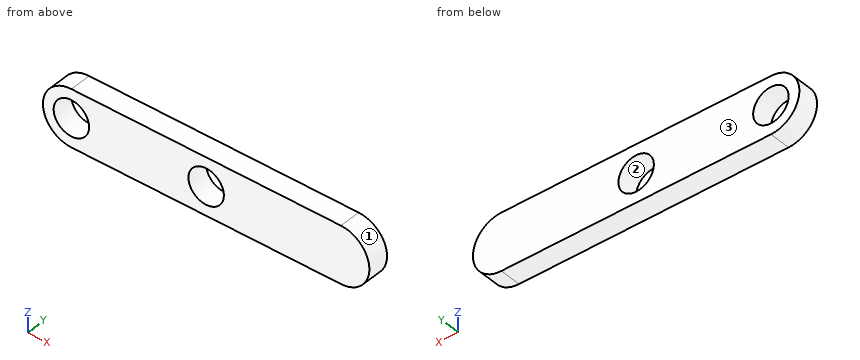
Autodesk Inventor part; units mm, degrees
ref_plane "YZ Plane" through (0, 0, 0) normal (1, 0, 0) x (0, 1, 0)
ref_plane "XZ Plane" through (0, 0, 0) normal (0, 1, 0) x (-1, 0, 0)
ref_plane "XY Plane" through (0, 0, 0) normal (0, 0, 1) x (1, 0, 0)
sketch "Sketch1" plane through (0, 0, 0) normal (0, 1, 0) x (-1, 0, 0)
  circle A0 centre (0, 0) radius 2.63
  line L0 (0, 0) -> (-2.63, 0) construction
  circle A1 centre (-20, 0) radius 2.63
  circle A2 centre (0, 0) radius 4.2175 construction
  circle A3 centre (-20, 0) radius 4.2175 construction
  line L1 (0, 4.2175) -> (-40, 4.2175)
  line L2 (0, -4.2175) -> (-40, -4.2175)
  arc A4 (-40, 4.2175) -> (-40, -4.2175) centre (-40, 0) ccw
  arc A5 (0, -4.2175) -> (0, 4.2175) centre (0, 0) ccw
  dimension "d0" = 5.26
  dimension "d1" = 20
  dimension "d2" = 1.5875
  dimension "d3" = 20
extrude "Extrusion1" add sketch "Sketch1" along normal blind 3.175
properties part number "CNC-011-XAxisHardStop" material "Aluminum 6061"
The listing builds one solid part. Answer for the finished solid, in the listing's coordinates (mm). Face numbers are marked on the shaded views. Round coordinates to 2 decimals unless told otherwise and drop trailing zeros. Loops run counter-clockwise (first coordinate to the right, second up) from the corner with the lowest first, then second, coordinate; pieces in that order, holes last. Notation, with made-up numbers: (-33, 84.5) - (10, 84.5) arc R11 cw to (10, 97.5) - close; hole circle Ø2 at (79.5, -31.75). An arc over 180 degrees is marked (long way). Return JSON: item names as keys, results as strings. Group by question number.
1. The part is cut by section A-A on x = 20. Determine the outline of the cut face in (y, z) (1 decimal).
2. The mould has two halves that part along Z. Classify the marked faces 1, 2 and 3: pulls with the +Z half, pulls with the -Z half, needs draft (parallel to the pull), parting line crosses it, or undercut.
3. This flat-tipped pin is pushed along its axis until it touches: P1, Ø1.5, axis at x = 14.5, z = 3, coming from the -Y side. Where does it stop, or does it pass through?
4. The part is cut by section D-D on z = -2. Determine the outline of the cut face in (x, y) (3 decimals).
5. The part is cut by section C-C on z = 1. Determine the outline of the cut face in (x, y) (3 decimals), then the cut area to 3 significant figures.
6. The part is cut by section B-B on y = 2.5. Determine the outline of the cut face in (x, z) (1 decimal).
7. Consider probe 1 along Z at (x, y) = (20, 1.2); probe 2 along X at (y, z) = (1.6, 0.75); probe 3 along X at (y, z) = (2.7, -1). Determine where each line is inside the solid, lowest interval first.
Resolved:
{
 "1": {"outline": "(0, -4.2) - (3.2, -4.2) - (3.2, -2.6) - (0, -2.6) - close; (0, 2.6) - (3.2, 2.6) - (3.2, 4.2) - (0, 4.2) - close"},
 "2": {"face 1": "parting line crosses it", "face 2": "undercut", "face 3": "needs draft"},
 "3": {"P1": "stops at y = 0"},
 "4": {"outline": "(-3.713, 0) - (-1.708, 0) - (-1.708, 3.175) - (-3.713, 3.175) - close; (1.708, 0) - (18.292, 0) - (18.292, 3.175) - (1.708, 3.175) - close; (21.708, 0) - (43.713, 0) - (43.713, 3.175) - (21.708, 3.175) - close"},
 "5": {"outline": "(-4.097, 0) - (-2.432, 0) - (-2.432, 3.175) - (-4.097, 3.175) - close; (2.432, 0) - (17.568, 0) - (17.568, 3.175) - (2.432, 3.175) - close; (22.432, 0) - (44.097, 0) - (44.097, 3.175) - (22.432, 3.175) - close", "area": "122 mm²"},
 "6": {"outline": "(0, -4.2) - (40, -4.2) arc R4.2 ccw to (40, 4.2) - (0, 4.2) arc R4.2 ccw to start; hole circle Ø5.3 at (0, 0); hole circle Ø5.3 at (20, 0)"},
 "7": {"probe 1": "z = -4.22 to -2.63, 2.63 to 4.22", "probe 2": "x = -4.15 to -2.52, 2.52 to 17.48, 22.52 to 44.15", "probe 3": "x = -4.1 to -2.43, 2.43 to 17.57, 22.43 to 44.1"}
}
